Check sheet for the drawn part. Datum: minimum x, y, z corner. Units: mm. A direction names the side the tool comes from. Round coordinates to 2 decimals unless told otherwise and drop trailing zeros. Loops run counter-clockwise (first coordinate to the right, second up) from the corner with the lowest first, then second, coordinate; pieces in that order, holes last. Notation, with made-up numbers: (2.25, 64) - (58.25, 64) arc R17 ccw to (58.25, 97) - close; hole circle Ø2 at (57, -38.75). An arc over 180 degrees is marked (long way). Use CSV: the item, a comma, the result in double quotes.
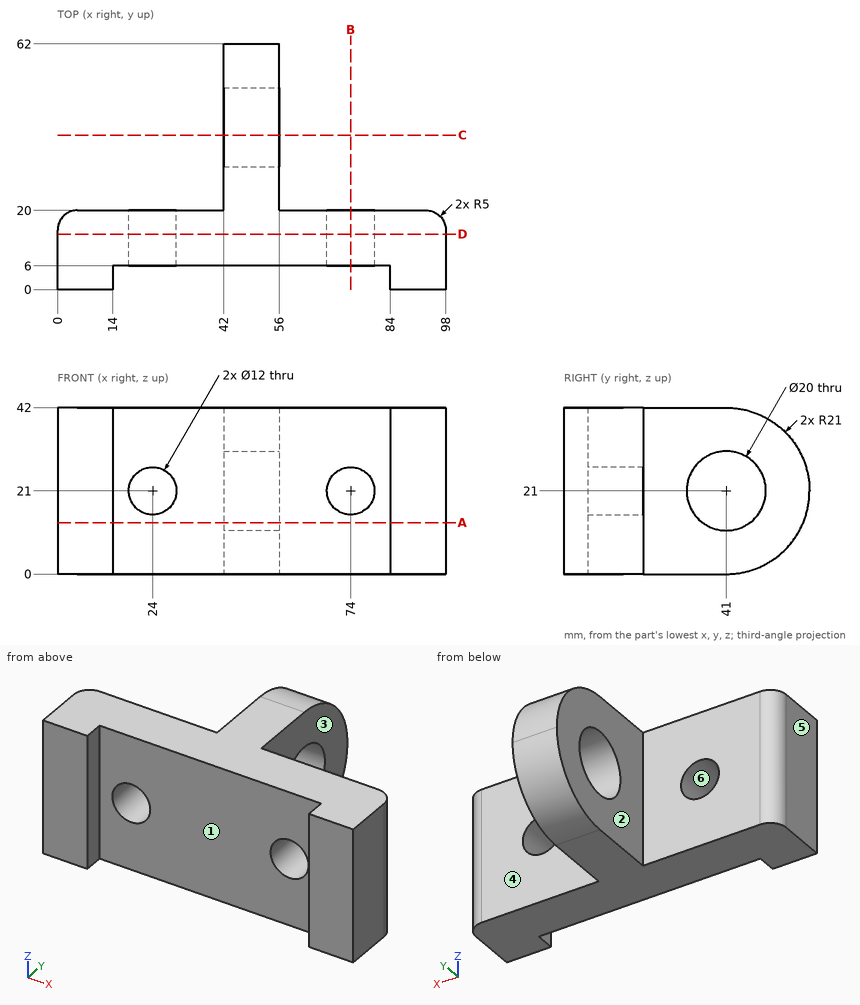
1) Cross-section at B-B, the plane x = 74. Record the cut outline in (y, z), then the cut area to 3 significant figures.
Returned:
outline,"(6, 0) - (20, 0) - (20, 15) - (6, 15) - close; (6, 27) - (20, 27) - (20, 42) - (6, 42) - close"
area,"420 mm²"
2) Mould release check, pull along X, two halves, no side actions. Record for the marked faces 4, 5 and 6: +X half, -X half, draft (parallel to the pull), parting line (faces both ways), or undercut.
Returned:
face 4,"draft"
face 5,"-X half"
face 6,"undercut"
3) Cross-section at D-D, the plane y = 14. Record the cut outline in (x, z).
Returned:
outline,"(0, 0) - (98, 0) - (98, 42) - (0, 42) - close; hole circle Ø12 at (24, 21); hole circle Ø12 at (74, 21)"
4) Cross-section at A-A, the plane z = 13. Record the cut outline in (x, y).
Returned:
outline,"(0, 0) - (14, 0) - (14, 6) - (84, 6) - (84, 0) - (98, 0) - (98, 15) arc R5 ccw to (93, 20) - (56, 20) - (56, 35) - (42, 35) - (42, 20) - (5, 20) arc R5 ccw to (0, 15) - close; (42, 47) - (56, 47) - (56, 60.42) - (42, 60.42) - close"
5) Thickness scan on probe 1 along Y at (x, z) = (49.5, 21); probe 2 along X at (y, z) = (10, 21); probe 3 along Y at (x, z) = (76, 31). Record the ranges inside material, lowest first. Write a range as [from, to].
Returned:
probe 1,"y = [6, 31], [51, 62]"
probe 2,"x = [0, 18], [30, 68], [80, 98]"
probe 3,"y = [6, 20]"
6) Cross-section at C-C, the plane y = 39. Record the cut outline in (x, z).
Returned:
outline,"(42, 0) - (56, 0) - (56, 11.2) - (42, 11.2) - close; (42, 30.8) - (56, 30.8) - (56, 42) - (42, 42) - close"
7) Gauge pin test, flat ends, axial feed: pin 1 Ø12 at (x, y) = (14, 20) entering from -Z; pin 2 Ø12 at (y, z) = (55.5, 36.5) entering from -X; pin 3 Ø3 at (y, z) = (17, 13.5) entering from +X (3 decimals); pin 4 Ø6 at (y, z) = (39, 16) entering from -X. Record the tip position at first contact, or that the pin passes through.
Returned:
pin 1,"stops at z = 0"
pin 2,"stops at x = 42"
pin 3,"stops at x = 97.975"
pin 4,"passes through"
8) Access from +Z, -Z, +X, -X, +Y, -Y to the whole of each face (thin tool, end or side, straight path). Record for the marked faces 1, 2 and 3.
Returned:
face 1,"+Z, -Z, -Y"
face 2,"+Z, -Z, -X, +Y"
face 3,"+Z, -Z, +X, +Y"
